Could you check a few things on this model? Use its own coordinates, in mm. Face numbers are marked on the shaded views. A direction names the side the tool comes from. Coordinates: 2 decimals unless noted, no trailing zeros. Loops run counter-clockwise (first coordinate to the right, second up) from the corner with the lowest first, then second, coordinate; pieces in that order, holes last. Notation, with made-up numbers: M 52.25,88 L 84.25,88 A32 cw 84.25,117 Z; hole C 72,-39.5 d11. An arc over 180 degrees is marked long. Write each question's results on one line, items separated by ' | '.
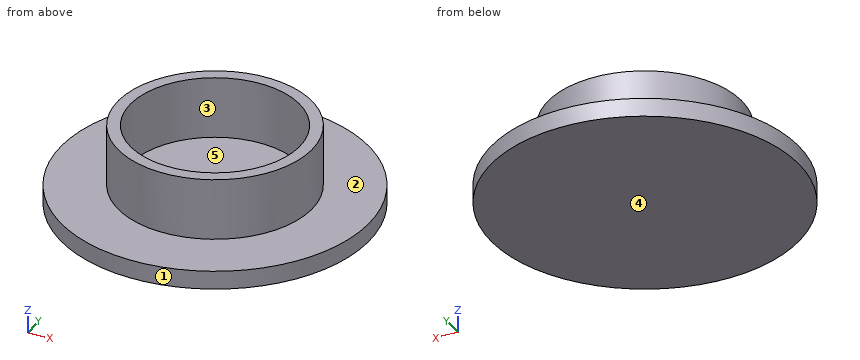
```python
from build123d import *

# Parameters (mm, degrees)
F0_R     = 25
F1_DEPTH = 3
F2_R     = 15.75
F3_DEPTH = 10
F4_R     = 13.75
F5_DEPTH = 10


with BuildPart() as f1:
    # F0 (on Top) → F1 (new body)
    with BuildSketch(Plane.XY):
        Circle(F0_R)
    extrude(amount=F1_DEPTH)

    # F2 (on face) → F3 (join)
    with BuildSketch(Plane.XY.offset(3)):
        Circle(F2_R)
    extrude(amount=F3_DEPTH)

    # F4 (on face) → F5 (cut, through all)
    with BuildSketch(Plane.XY.offset(13)):
        Circle(F4_R)
    extrude(amount=-F5_DEPTH, mode=Mode.SUBTRACT)


solid = f1.part
```
(1) Imagine slicing it at C-C, the plane z = 10.5. List the corners of the cut face in (x, y) for me.
Reported:
outline: C 0,0 d31.5; hole C 0,0 d27.5
(2) Imagine slicing it at A-A, the plane x = 0. List the corners of the cut face in (y, z) for me.
Reported:
outline: M -25,0 L 25,0 L 25,3 L 15.75,3 L 15.75,13 L 13.75,13 L 13.75,3 L -13.75,3 L -13.75,13 L -15.75,13 L -15.75,3 L -25,3 Z
(3) If we mould it in two halves opening along Y, with no side actions, what happens to the marked faces 1, 2 and 3? For each: released by +Y, released by -Y, zero draft, split by the parting line, or undercut.
Reported:
face 1: split by the parting line | face 2: zero draft | face 3: undercut
(4) Imagine slicing it at D-D, the plane z = 2.25. List the corners of the cut face in (x, y) for me, and give its area (3 significant figures).
Reported:
outline: C 0,0 d50 | area: 1,960 mm2
(5) Which directions (+Z, -Z, +X, -X, +Y, -Y) give clear straight access to the entire face, cutting with the end or side of a thin tool? Please do the marked faces 4 and 5.
Reported:
face 4: -Z, +X, -X, +Y, -Y | face 5: +Z
(6) Please list where these lines run through material, in increasing order: probe 1 along Y at (x, z) = (0, 10.25); probe 2 along Z at (x, y) = (1, -19.5); probe 3 along Y at (x, z) = (-11.5, 4.75). Write a range as from..to.
Reported:
probe 1: y = -15.75..-13.75, 13.75..15.75 | probe 2: z = 0..3 | probe 3: y = -10.76..-7.54, 7.54..10.76
(7) Will these pins go through, and if not, where does the flat tip stop? P1, Ø1, axis at x = -14, y = 13, coming from the +Z side; P2, Ø2, axis at x = 12.5, z = 10, coming from the +Y side; P3, Ø6, axis at x = 8.5, z = 11, coming from the +Y side; P4, Ø4, axis at x = -19, z = 6.5, coming from the -Y side.
Reported:
P1: stops at z = 3 | P2: stops at y = 10.76 | P3: stops at y = 14.76 | P4: passes through
